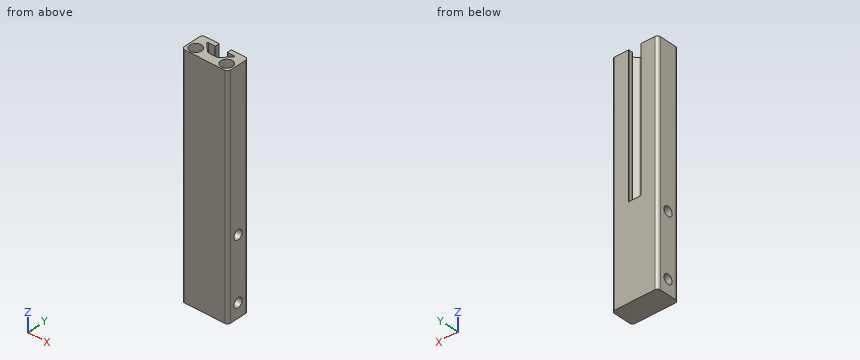
from build123d import *

# Parameters (mm, degrees)
SKETCH3_R                  = 3.2385
BOSS_EXTRUDE1_DEPTH        = 38.1
FILLET1_R                  = 0.254
BOSS_EXTRUDE2_DEPTH        = 50.8
F_8_0_199_DIAMETER_HOLE8_D = 5.0546
LPATTERN1_COUNT            = 2
LPATTERN1_PITCH            = 34.036


with BuildPart() as part:
    # Sketch3 → Boss-Extrude1 (new body, symmetric)
    with BuildSketch(Plane.XY):
        with BuildLine():
            Line((-11.049, 12.7), (-3.302, 12.7))
            Line((-3.302, 12.7), (-3.302, 10.328863887))
            Line((-3.302, 10.328863887), (-6.985, 10.328863887))
            ThreePointArc((-6.985, 10.328863887), (-7.454330803, 10.01526707), (-7.344210245, 9.461653642))
            Line((-7.344210245, 9.461653642), (-3.452505379, 5.569948776))
            ThreePointArc((-3.452505379, 5.569948776), (-2.628470073, 5.019345987), (-1.656454155, 4.826))
            Line((-1.656454155, 4.826), (1.656454155, 4.826))
            ThreePointArc((1.656454155, 4.826), (2.628470073, 5.019345987), (3.452505379, 5.569948776))
            Line((3.452505379, 5.569948776), (7.344210245, 9.461653642))
            ThreePointArc((7.344210245, 9.461653642), (7.454330803, 10.01526707), (6.985, 10.328863887))
            Line((6.985, 10.328863887), (3.302, 10.328863887))
            Line((3.302, 10.328863887), (3.302, 12.7))
            Line((3.302, 12.7), (11.049, 12.7))
            ThreePointArc((11.049, 12.7), (12.216433296, 12.216433296), (12.7, 11.049))
            Line((12.7, 11.049), (12.7, 1.651))
            ThreePointArc((12.7, 1.651), (12.216433296, 0.483566704), (11.049, 0))
            Line((11.049, 0), (-11.049, 0))
            ThreePointArc((-11.049, 0), (-12.216433296, 0.483566704), (-12.7, 1.651))
            Line((-12.7, 1.651), (-12.7, 11.049))
            ThreePointArc((-12.7, 11.049), (-12.216433296, 12.216433296), (-11.049, 12.7))
        make_face()
        with Locations((8.509, 4.064)):
            Circle(SKETCH3_R, mode=Mode.SUBTRACT)
        with Locations((-8.509, 4.064)):
            Circle(SKETCH3_R, mode=Mode.SUBTRACT)
    extrude(amount=BOSS_EXTRUDE1_DEPTH, both=True)

    # Fillet1
    fillet1_edges = [part.edges().sort_by_distance(p)[0] for p in [
        (-3.302, 12.7, 0),
        (-3.302, 10.328863887, 0),
        (3.302, 10.328863887, 0),
        (3.302, 12.7, 0),
    ]]
    fillet(fillet1_edges, radius=FILLET1_R)

    # Sketch4 → Boss-Extrude2 (add)
    with BuildSketch(Plane(origin=(0, 0, -38.1), x_dir=(-1, 0, 0), z_dir=(0, 0, -1))):
        with BuildLine():
            Line((3.556, 12.7), (-11.049, 12.7))
            ThreePointArc((-11.049, 12.7), (-12.216433296, 12.216433296), (-12.7, 11.049))
            Line((-12.7, 11.049), (-12.7, 1.651))
            ThreePointArc((-12.7, 1.651), (-12.216433296, 0.483566704), (-11.049, 0))
            Line((-11.049, 0), (11.049, 0))
            ThreePointArc((11.049, 0), (12.216433296, 0.483566704), (12.7, 1.651))
            Line((12.7, 1.651), (12.7, 11.049))
            ThreePointArc((12.7, 11.049), (12.216433296, 12.216433296), (11.049, 12.7))
            Line((11.049, 12.7), (3.556, 12.7))
        make_face()
    extrude(amount=BOSS_EXTRUDE2_DEPTH)

    # #8 (0.199) Diameter Hole8 (through all)
    with Locations(Plane(origin=(12.7, 0, 0), x_dir=(0, 0, -1), z_dir=(1, 0, 0))):
        with Locations((81.026, 6.35)):
            f_8_0_199_diameter_hole8 = Hole(F_8_0_199_DIAMETER_HOLE8_D / 2)

    # LPattern1: #8 (0.199) Diameter Hole8 ×2
    with Locations(*[(0, 0, i * LPATTERN1_PITCH) for i in range(1, LPATTERN1_COUNT)]):
        add(f_8_0_199_diameter_hole8, mode=Mode.SUBTRACT)


solid = part.part
Could you check a few things on this model? Use its own coordinates, in mm. Coordinates: 2 decimals unless noted, no trailing zeros. Write each loop counter-clockwise with the first axis right and the second up, starting at its lowest first coordinate (ties: lowest second). Pieces come first, ordered by that corner, then holes. Notation, with made-up numbers: (-15, 82.5) - (-9, 82.5) arc R18 ccw to (-9, 88.5) - close; hole circle Ø4 at (-13, 86.5). An arc over 180 degrees is marked (long way). Put each result on its own line as item: value. Start each with the question number.
Q1. I want a section at D-D on x = 9.25. Write out the boundary of the cut face in (y, z), plus the area to 3 significant figures.
Q2. I want a section at B-B on z = -46.99. Write out the boundary of the cut face in (x, y), plus the area to 3 significant figures.
Q3. I want a section at A-A on x = 0.5. Write out the boundary of the cut face in (y, z).
Q4. Please list where these lines run through material, in increasing order: L1, parallel to Z at x = 7.5, y = 6; L2, parallel to X at y = 2.5, z = -18; L3, parallel to X at y = 9.75, z = -7.
Q5. I want a section at C-C on z = -6.5. Count the separate pieces of the cut face and the enclosed holes in it, plus the area to 3 significant figures.
Q6. I'm going to push flat-ended pins straight in: P1, Ø4, axis at x = 8.509, y = 4.064, coming from the +Z side; P2, Ø6, axis at y = 6.35, z = -46.99, coming from the -X side; P3, Ø3.5, axis at x = 0, z = 17, coming from the +Y side. Where does each tip first touch, or does it pass through?
Checks:
1. outline: (0, -88.9) - (12.7, -88.9) - (12.7, 38.1) - (7.22, 38.1) - (7.22, -38.1) - (0.91, -38.1) - (0.91, 38.1) - (0, 38.1) - close; hole circle Ø5.05 at (6.35, -81.03); hole circle Ø5.05 at (6.35, -46.99)
1. area: 1,090 mm²
2. outline: (-12.7, 1.65) arc R1.65 ccw to (-11.05, 0) - (11.05, 0) arc R1.65 ccw to (12.7, 1.65) - (12.7, 3.82) - (-12.7, 3.82) - close; (-12.7, 8.88) - (12.7, 8.88) - (12.7, 11.05) arc R1.65 ccw to (11.05, 12.7) - (-11.05, 12.7) arc R1.65 ccw to (-12.7, 11.05) - close
2. area: 192 mm²
3. outline: (0, -88.9) - (12.7, -88.9) - (12.7, -38.1) - (4.83, -38.1) - (4.83, 38.1) - (0, 38.1) - close; hole circle Ø5.05 at (6.35, -81.03); hole circle Ø5.05 at (6.35, -46.99)
4. L1: -88.9 to -83.53, -78.52 to -49.49, -44.49 to -38.1
4. L2: -12.7 to -11.34, -5.67 to 5.67, 11.34 to 12.7
4. L3: -12.7 to -7.49, 7.49 to 12.7
5. separate pieces: 1
5. enclosed holes: 2
5. area: 179 mm²
6. P1: z = -38.1
6. P2: x = -12.7
6. P3: y = 4.83
